For this review, take the finished solid that the model builds, in its own axes (mm). Face numbers are marked on the shaded views. A direction names the side the tool comes from. Round coordinates to 2 decimals unless told otherwise and drop trailing zeros. Order: outer loops, then holes, each group sorted by start corner. A loop starts at its lowest first (then second) coordinate and runs counter-clockwise, first axis right, second up. Notation, with made-up numbers: (-10, 3.5) - (42, 3.5) arc R23 ccw to (42, 19.5) - close; hole circle Ø6 at (62, -39). An arc over 180 degrees is marked (long way). One line per item, written item: value.
```python
from build123d import *

# Parameters (mm, degrees)
SKETCH1_W            = 303
SKETCH1_H            = 350
BASE_FLANGE1_DEPTH   = 2
EDGE_FLANGE1_DEPTH   = 350
CUT_EXTRUDE1_REACH   = 468.294
CUT_EXTRUDE2_REACH   = 468.294
LPATTERN1_COUNT      = 2
LPATTERN1_PITCH      = 100
MIRROR1_COPY_1_REACH = 468.294


# Sheet-metal steps are written as plain solids
with BuildPart() as part:
    # Sketch1 → Base-Flange1 (new body)
    with BuildSketch(Plane.XY):
        with Locations((-151.5, 175)):
            Rectangle(SKETCH1_W, SKETCH1_H)
    extrude(amount=-BASE_FLANGE1_DEPTH)

    # Edge-Flange1 section (across the edge) → Edge-Flange1 (add)
    with BuildSketch(Plane(origin=(-303.5, 0, -2), x_dir=(1, 0, 0), z_dir=(0, 1, 0))):
        with BuildLine():
            Line((-2, 0.5), (-2, 38))
            Line((-2, 38), (0, 38))
            Line((0, 38), (0, 0.5))
            ThreePointArc((0, 0.5), (0.146446609, 0.146446609), (0.5, 0))
            Line((0.5, 0), (0.5, -2))
            ThreePointArc((0.5, -2), (-1.267766953, -1.267766953), (-2, 0.5))
        make_face()
    edge_flange1 = extrude(amount=EDGE_FLANGE1_DEPTH)

    # Sketch15 → Cut-Extrude1 (cut, up to next)
    with BuildSketch(Plane.ZY.offset(305.5), mode=Mode.PRIVATE) as cut_extrude1_sk1:
        Polygon((-2.5, 0), (-2.5, 121), (-40, 142.650635095), (-40, 0), align=None)
    cut_extrude1_tool1 = extrude(cut_extrude1_sk1.sketch, amount=-CUT_EXTRUDE1_REACH, mode=Mode.PRIVATE) & part.part
    cut_extrude1 = cut_extrude1_tool1.solids().sort_by_distance((-305.5, 66.060819, -21.763242))[0]
    add(cut_extrude1, mode=Mode.SUBTRACT)

    # Sketch18 → Cut-Extrude2 (cut, up to next)
    with BuildSketch(Plane.ZY.offset(305.5), mode=Mode.PRIVATE) as cut_extrude2_sk1:
        with BuildLine():
            Line((-29.6559, 235.1372), (-29.6559, 205.1372))
            ThreePointArc((-29.6559, 205.1372), (-31.3559, 203.4372), (-33.0559, 205.1372))
            Line((-33.0559, 205.1372), (-33.0559, 235.1372))
            ThreePointArc((-33.0559, 235.1372), (-31.3559, 236.8372), (-29.6559, 235.1372))
        make_face()
    cut_extrude2_tool1 = extrude(cut_extrude2_sk1.sketch, amount=-CUT_EXTRUDE2_REACH, mode=Mode.PRIVATE) & part.part
    cut_extrude2 = cut_extrude2_tool1.solids().sort_by_distance((-305.5, 220.1372, -31.3559))[0]
    add(cut_extrude2, mode=Mode.SUBTRACT)

    # LPattern1: Cut-Extrude2 ×2
    with Locations(*[(0, i * LPATTERN1_PITCH, 0) for i in range(1, LPATTERN1_COUNT)]):
        add(cut_extrude2, mode=Mode.SUBTRACT)

    # Mirror1: Edge-Flange1, Cut-Extrude1, Cut-Extrude2 across plane
    add(edge_flange1.mirror(Plane.ZY.offset(151.5)))
    add(cut_extrude1.mirror(Plane.ZY.offset(151.5)), mode=Mode.SUBTRACT)
    add(cut_extrude2.mirror(Plane.ZY.offset(151.5)), mode=Mode.SUBTRACT)

    # Mirror1 copy 1 sketch → Mirror1 copy 1 (cut, up to next)
    with BuildSketch(Plane(origin=(2.5, 100, 0), x_dir=(0, 0, 1), z_dir=(1, 0, 0)), mode=Mode.PRIVATE) as mirror1_copy_1_sk1:
        with BuildLine():
            Line((-29.6559, -235.1372), (-29.6559, -205.1372))
            ThreePointArc((-29.6559, -205.1372), (-31.3559, -203.4372), (-33.0559, -205.1372))
            Line((-33.0559, -205.1372), (-33.0559, -235.1372))
            ThreePointArc((-33.0559, -235.1372), (-31.3559, -236.8372), (-29.6559, -235.1372))
        make_face()
    mirror1_copy_1_tool1 = extrude(mirror1_copy_1_sk1.sketch, amount=-MIRROR1_COPY_1_REACH, mode=Mode.PRIVATE) & part.part
    add(mirror1_copy_1_tool1.solids().sort_by_distance((2.5, 320.1372, -31.3559))[0], mode=Mode.SUBTRACT)


solid = part.part
```
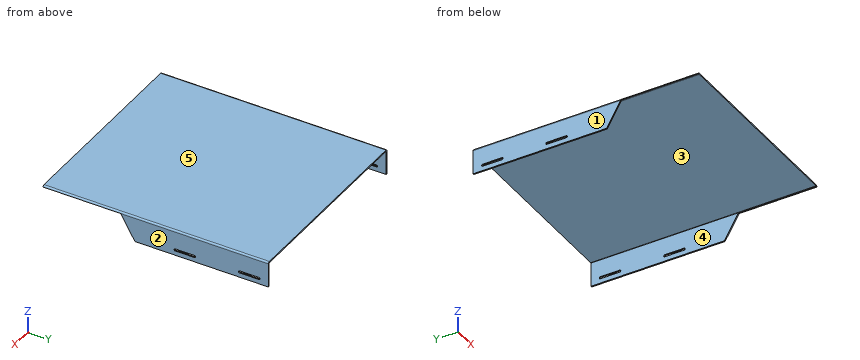
Item 1: Take a section at B-B (z = -25). Write out the cut boundary in (x, y), plus the area to 3 significant figures.
Returned:
outline: (-305.5, 133.99) - (-303.5, 133.99) - (-303.5, 350) - (-305.5, 350) - close; (0.5, 133.99) - (2.5, 133.99) - (2.5, 350) - (0.5, 350) - close
area: 864 mm^2
Item 2: Take a section at D-D (z = -7.5). Write out the cut boundary in (x, y), plus the area to 3 significant figures.
Returned:
outline: (-305.5, 123.89) - (-303.5, 123.89) - (-303.5, 350) - (-305.5, 350) - close; (0.5, 123.89) - (2.5, 123.89) - (2.5, 350) - (0.5, 350) - close
area: 904 mm^2
Item 3: Take a section at A-A (y = 228.5). Write out the cut boundary in (x, z).
Returned:
outline: (-305.5, -40) - (-303.5, -40) - (-303.5, -33.06) - (-305.5, -33.06) - close; (-305.5, -29.66) - (-303.5, -29.66) - (-303.5, -2.5) arc R0.5 cw to (-303, -2) - (0, -2) arc R0.5 cw to (0.5, -2.5) - (0.5, -29.66) - (2.5, -29.66) - (2.5, -2.5) arc R2.5 ccw to (0, 0) - (-303, 0) arc R2.5 ccw to (-305.5, -2.5) - close; (0.5, -40) - (2.5, -40) - (2.5, -33.06) - (0.5, -33.06) - close
Item 4: The part is to be moulded in two halves that separate along X. For the marked faces 1, 2 and 3, say which applies: +X half, -X half, draft (parallel to the pull), parting line (faces both ways), or undercut.
Returned:
face 1: -X half
face 2: +X half
face 3: undercut
Item 5: For P1, Ø4, axis at x = -42.5, y = 121, coming from the +Z side; P2, Ø1.6, axis at x = -304.5, y = 313.5, coming from the +Z side; P3, Ø1.6, axis at x = 1.5, y = 85.5, coming from the -Z side; P4, Ø4, axis at x = -122, y = 292, coming from the -Z side, all flat-tipped, find the tip position at first contact; note any pin that passes through.
Returned:
P1: z = 0
P2: z = -0.1
P3: z = -2.5
P4: z = -2
Item 6: Take a section at C-C (y = 267.5). Write out the cut boundary in (x, z), plus the area to 3 significant figures.
Returned:
outline: (-305.5, -40) - (-303.5, -40) - (-303.5, -2.5) arc R0.5 cw to (-303, -2) - (0, -2) arc R0.5 cw to (0.5, -2.5) - (0.5, -40) - (2.5, -40) - (2.5, -2.5) arc R2.5 ccw to (0, 0) - (-303, 0) arc R2.5 ccw to (-305.5, -2.5) - close
area: 765 mm^2
Item 7: Wall thickness on line 1 (X direction, y = 151, z = -32); line 2 (Z direction, x = -125, y = 284.5): over which ranges is each line inside the solid? List them lowest first.
Returned:
line 1: -305.5 to -303.5, 0.5 to 2.5
line 2: -2 to 0
Item 8: Machinability: for the marked faces 4 and 5, which of the approach directions +Z, -Z, +X, -X, +Y, -Y give a long, thin tool a straight path to every point of the face, cutting with its end or side? Answer none if there is none.
Returned:
face 4: -Z, +Y, -Y
face 5: +Z, +X, -X, +Y, -Y
